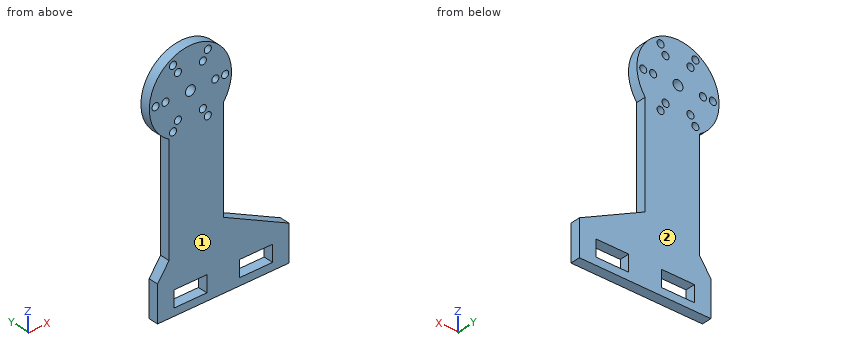
```python
from build123d import *

# Parameters (mm, degrees)
SKETCH_1_R      = 1.075
SKETCH_1_R_2    = 1.5
SKETCH_1_W      = 10
SKETCH_1_H      = 5
EXTRUDE_2_DEPTH = 3


with BuildPart() as part:
    # 草图1 → 凸台-拉伸2 (new body)
    with BuildSketch(Plane(origin=(0, 0, 0), x_dir=(1, 0, 0), z_dir=(0, 1, 0))):
        with BuildLine():
            Line((-6.5, 10.677078252), (-6.5, 44.1))
            Line((-6.5, 44.1), (-10, 49.098518024))
            Line((-10, 49.098518024), (-10, 60.1))
            Line((-10, 60.1), (30, 60.1))
            Line((30, 60.1), (30, 49.1))
            Line((30, 49.1), (10, 39.1))
            Line((10, 39.1), (10, 7.5))
            ThreePointArc((10, 7.5), (-2.363462831, -12.274528237), (-6.5, 10.677078252))
        make_face()
        with Locations(Location((7.58, 0, 0), (0, 0, 270))):
            Circle(SKETCH_1_R, mode=Mode.SUBTRACT)
        with Locations(Location((10.58, 0, 0), (0, 0, 270))):
            Circle(SKETCH_1_R, mode=Mode.SUBTRACT)
        with Locations(Location((3.79, -6.564472561, 0), (0, 0, 270))):
            Circle(SKETCH_1_R, mode=Mode.SUBTRACT)
        with Locations(Location((5.29, -9.162548772, 0), (0, 0, 270))):
            Circle(SKETCH_1_R, mode=Mode.SUBTRACT)
        with Locations(Location((-3.79, -6.564472561, 0), (0, 0, 270))):
            Circle(SKETCH_1_R, mode=Mode.SUBTRACT)
        with Locations(Location((-5.29, -9.162548772, 0), (0, 0, 270))):
            Circle(SKETCH_1_R, mode=Mode.SUBTRACT)
        with Locations(Location((-7.58, 0, 0), (0, 0, 270))):
            Circle(SKETCH_1_R, mode=Mode.SUBTRACT)
        with Locations(Location((-10.58, 0, 0), (0, 0, 270))):
            Circle(SKETCH_1_R, mode=Mode.SUBTRACT)
        with Locations(Location((-3.79, 6.564472561, 0), (0, 0, 270))):
            Circle(SKETCH_1_R, mode=Mode.SUBTRACT)
        with Locations(Location((-5.29, 9.162548772, 0), (0, 0, 270))):
            Circle(SKETCH_1_R, mode=Mode.SUBTRACT)
        with Locations(Location((3.79, 6.564472561, 0), (0, 0, 270))):
            Circle(SKETCH_1_R, mode=Mode.SUBTRACT)
        with Locations(Location((5.29, 9.162548772, 0), (0, 0, 270))):
            Circle(SKETCH_1_R, mode=Mode.SUBTRACT)
        with Locations(Location((0, 0, 0), (0, 0, 270))):
            Circle(SKETCH_1_R_2, mode=Mode.SUBTRACT)
        with Locations((0, 55.314192659)):
            Rectangle(SKETCH_1_W, SKETCH_1_H, mode=Mode.SUBTRACT)
        with Locations((20, 55.314192659)):
            Rectangle(SKETCH_1_W, SKETCH_1_H, mode=Mode.SUBTRACT)
    extrude(amount=EXTRUDE_2_DEPTH)


solid = part.part
```
Source: CAD feature listing. Evaluate the final solid. Frame: model axes, mm. Face numbers are marked on the shaded views. Round coordinates to 2 decimals unless told otherwise and drop trailing zeros. Loops run counter-clockwise (first coordinate to the right, second up) from the corner with the lowest first, then second, coordinate; pieces in that order, holes last.
1. Ray query, L1, parallel to X at y = 2.45, z = 0 (3 decimals); L2, parallel to X at y = 2.15, z = -55; L3, parallel to X at y = 2.6, z = -10. Return the intervals inside material, ascending.
2. Contact query for flat-ended pins moving along their axis: pin 1 (1.3 mm diameter, centred on x = 7.58, z = 0, fed in from +Y); pin 2 (1.5 mm diameter, centred on x = 2, y = 2, fed in from +Z); pin 3 (0.9 mm diameter, centred on y = 1, z = -55, fed in from -X). Output: stop coordinate, or through.
3. Section query A-A on x = 0. Output: boundary loops of the cut face in (y, z), and give its area (3 significant figures).
4. Section query D-D on x = 22.5. Output: boundary loops of the cut face in (y, z).
5. Mould query, pull axis Y, two halves, no side actions, for the marked faces 1 and 2. Classes: released by +Y, released by -Y, zero draft, split by the parting line, or undercut.
6. Section query B-B on y = 1.5. Give the number of separate pieces and of enclosed holes in the cut face, and give its area (3 significant figures).
7. Section query C-C on z = 0. Output: boundary loops of the cut face in (x, y) (3 decimals).
Answers below:
1. L1: x = -12.5 to -11.655, -9.505 to -8.655, -6.505 to -1.5, 1.5 to 6.505, 8.655 to 9.505, 11.655 to 12.5
1. L2: x = -10 to -5, 5 to 15, 25 to 30
1. L3: x = -7.5 to -5.96, -4.62 to 4.62, 5.96 to 10
2. pin 1: passes through
2. pin 2: stops at z = 12.44
2. pin 3: stops at x = -10
3. outline: (0, -60.1) - (3, -60.1) - (3, -57.81) - (0, -57.81) - close; (0, -52.81) - (3, -52.81) - (3, -1.5) - (0, -1.5) - close; (0, 1.5) - (3, 1.5) - (3, 12.5) - (0, 12.5) - close
3. area: 194 mm2
4. outline: (0, -60.1) - (3, -60.1) - (3, -57.81) - (0, -57.81) - close; (0, -52.81) - (3, -52.81) - (3, -45.35) - (0, -45.35) - close
5. face 1: released by -Y
5. face 2: released by +Y
6. separate pieces: 1
6. enclosed holes: 15
6. area: 1,510 mm2
7. outline: (-12.5, 0) - (-11.655, 0) - (-11.655, 3) - (-12.5, 3) - close; (-9.505, 0) - (-8.655, 0) - (-8.655, 3) - (-9.505, 3) - close; (-6.505, 0) - (-1.5, 0) - (-1.5, 3) - (-6.505, 3) - close; (1.5, 0) - (6.505, 0) - (6.505, 3) - (1.5, 3) - close; (8.655, 0) - (9.505, 0) - (9.505, 3) - (8.655, 3) - close; (11.655, 0) - (12.5, 0) - (12.5, 3) - (11.655, 3) - close
